from build123d import *

# Parameters (mm, degrees)
CROQUIS1_W              = 8
CROQUIS1_H              = 5
SALIENTE_EXTRUIR1_DEPTH = 4
CROQUIS2_W              = 8
CROQUIS2_H              = 1.5
CORTAR_EXTRUIR1_DEPTH   = 1.5
CROQUIS3_W              = 8
CROQUIS3_H              = 5
SALIENTE_EXTRUIR2_DEPTH = 4
REDONDEO1_R             = 10


with BuildPart() as part:
    # Croquis1 → Saliente-Extruir1 (new body)
    with BuildSketch(Plane.XY):
        Rectangle(CROQUIS1_W, CROQUIS1_H)
    extrude(amount=SALIENTE_EXTRUIR1_DEPTH)

    # Croquis2 → Cortar-Extruir1 (cut)
    with BuildSketch(Plane.XY.offset(4)):
        Rectangle(CROQUIS2_W, CROQUIS2_H)
    extrude(amount=-CORTAR_EXTRUIR1_DEPTH, mode=Mode.SUBTRACT)

    # Croquis3 → Saliente-Extruir2 (add)
    with BuildSketch(Plane.XY.offset(4)):
        with BuildLine():
            Line((-4, 2.5), (4, 2.5))
            ThreePointArc((4, 2.5), (0, 2.792464279), (-4, 2.5))
        make_face()
        with Locations((0, -3.25)):
            Rectangle(CROQUIS3_W, CROQUIS3_H)
    extrude(amount=-SALIENTE_EXTRUIR2_DEPTH)

    # Redondeo1
    # the kernel refuses this fillet: 10 mm, written as the material it takes off along each edge
    with BuildSketch(Plane(origin=(24, -5.75, 0), x_dir=(0, 0, 1), z_dir=(-1, 0, 0))) as redondeo1_piece_1:
        with BuildLine():
            CenterArc((10, 8), REDONDEO1_R, 180, 53.130102354)
            Line((0, 8), (-0.2, 8))
            Line((-0.2, 8), (-0.2, 0))
            Line((-0.2, 0), (0, -0.2))
            ThreePointArc((0, -0.2), (2, -0.2), (3.88, -0.16))
            Line((3.88, -0.16), (4, 0))
        make_face()
    extrude(amount=48, mode=Mode.SUBTRACT)


solid = part.part
Work out the finished part from the listing and answer in its coordinate system (mm). A direction names the side the tool comes from. Round coordinates to 2 decimals unless told otherwise and drop trailing zeros. Write each loop counter-clockwise with the first axis right and the second up, starting at its lowest first coordinate (ties: lowest second). Pieces come first, ordered by that corner, then holes.
1) Given pin 1 Ø1.6 at (x, z) = (2, 3) entering from +Y; pin 2 Ø0.8 at (x, y) = (-1.5, 0) entering from +Z; pin 3 Ø1.5 at (x, y) = (3, -3) entering from -Z, each flat-ended and moving along its own axis, determine where each tip first touches the part or whether it passes through.
2) Straight lines are drawn through the part: line 1 (Z direction, x = 0.5, y = 2); line 2 (Y direction, x = -3, z = 3.3); line 3 (Y direction, x = 0.25, z = 3.2). For each, find the intervals that lie inside material, in ascending order.
3) The mould has two halves that part along Y. Classify faces 3 (the flat face through (0, -0.75, 3)), 4 (the cylindrical face through (0.056, -2.164, 1.027)), 5 (the flat face through (0, 0, 2.5)), 6 (the flat face through (0, 2, 4)): pulls with the +Y half, pulls with the -Y half, needs draft (parallel to the pull), parting line crosses it, or undercut.
4) A cutting plane is placed at A-A (x = 0). Give the vertices of the cut face in (y, z), plus the area to 3 significant figures.
5) A cutting plane is placed at C-C (z = 3.3). Give the vertices of the cut face in (x, y).
6) A tool of negligible diameter and unlimited length cuts with its end or side. For faces 1 (the cylindrical face through (0.056, 2.792, 2.028)), 2 (the flat face through (0, 0.75, 3)), from which of +Z, -Z, +X, -X, +Y, -Y can it reach the whole face along a straight path? Write none if from no direction.
7) A cutting plane is placed at B-B (z = 3.75). Give the vertices of the cut face in (x, y).
8) A cutting plane is placed at D-D (y = -4.75). Give the vertices of the cut face in (x, z), plus the area to 3 significant figures.
Completed:
1. pin 1: stops at y = 2.77
1. pin 2: stops at z = 2.5
1. pin 3: stops at z = 1.07
2. line 1: z = 0 to 4
2. line 2: y = -5.17 to -0.75, 0.75 to 2.63
2. line 3: y = -5.08 to -0.75, 0.75 to 2.79
3. face 3: undercut
3. face 4: pulls with the -Y half
3. face 5: undercut
3. face 6: needs draft
4. outline: (-5.75, 4) arc R10 ccw to (2.25, 0) - (2.79, 0) - (2.79, 4) - (0.75, 4) - (0.75, 2.5) - (-0.75, 2.5) - (-0.75, 4) - close
4. area: 22.3 mm2
5. outline: (-4, -5.17) - (4, -5.17) - (4, -0.75) - (-4, -0.75) - close; (-4, 0.75) - (4, 0.75) - (4, 2.5) arc R27.5 ccw to (-4, 2.5) - close
6. face 1: +Z, -Z, +Y
6. face 2: +Z, +X, -X
7. outline: (-4, -5.56) - (4, -5.56) - (4, -0.75) - (-4, -0.75) - close; (-4, 0.75) - (4, 0.75) - (4, 2.5) arc R27.5 ccw to (-4, 2.5) - close
8. outline: (-4, 2.86) - (4, 2.86) - (4, 4) - (-4, 4) - close
8. area: 9.13 mm2
